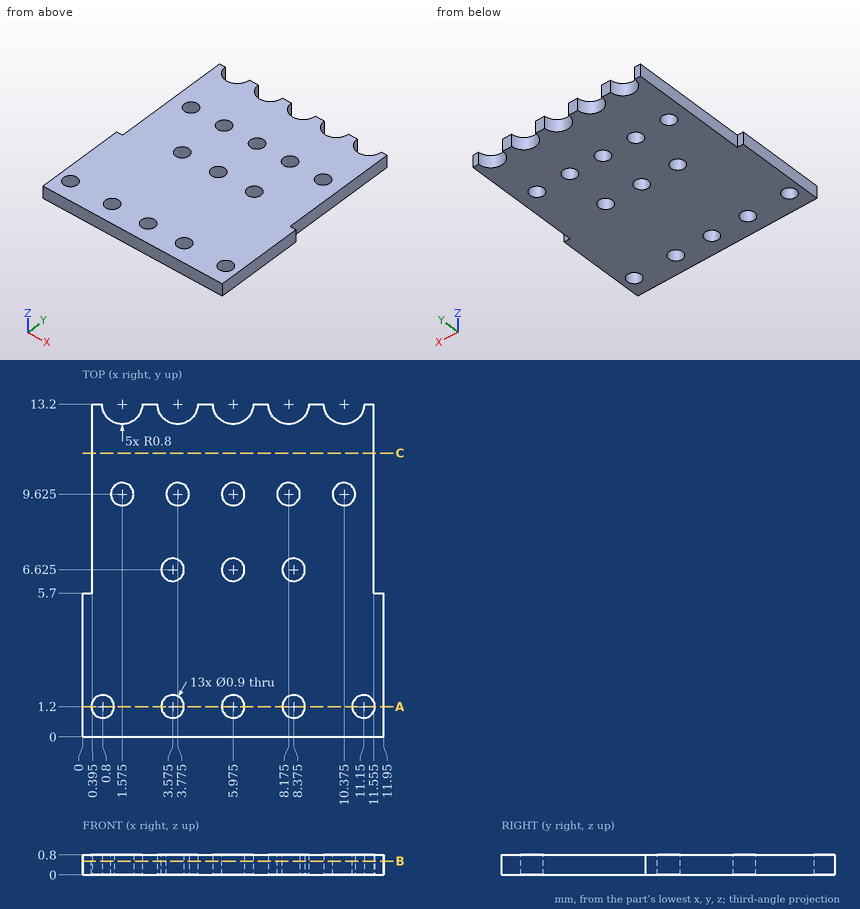
Could you check a few things on this drawing? It's one solid part, dimensions in mm from its lowest x, y, z. Round coordinates to 2 decimals unless told otherwise and drop trailing zeros. Order: outer loops, then holes, each group sorted by start corner. A loop starts at its lowest first (then second) coordinate and runs counter-clockwise, first axis right, second up. Notation, with made-up numbers: M -14,43.25 L -2,43.25 A19 ccw -2,51.25 Z; hole C 19.5,37 d11. An arc over 180 degrees is marked long. Return JSON: item names as keys, results as strings. Group by question number.
1. Please list where these lines run through material, in increasing order: probe 1 along Y at (x, z) = (6, 0.3); probe 2 along Y at (x, z) = (3.25, 0.35); probe 3 along X at (y, z) = (6.25, 0.2) (3 decimals).
2. If we section it at A-A on y = 1.2: List the corners of the cut face in (x, z) for me (3 decimals), then the cut area to 3 significant figures.
3. If we section it at B-B on z = 0.55: State how many separate pieces and enclosed holes the cut face has, then the cut area to 3 significant figures.
4. If we section it at C-C on y = 11.25: List the corners of the cut face in (x, z) for me (3 decimals).
Reply:
{
 "1": {"probe 1": "0 to 0.75, 1.65 to 6.18, 7.07 to 9.18, 10.07 to 12.4", "probe 2": "0 to 0.89, 1.51 to 6.31, 6.94 to 12.6", "probe 3": "0.395 to 3.326, 3.824 to 5.726, 6.224 to 8.126, 8.624 to 11.555"},
 "2": {"outline": "M 0,0 L 0.35,0 L 0.35,0.8 L 0,0.8 Z; M 1.25,0 L 3.125,0 L 3.125,0.8 L 1.25,0.8 Z; M 4.025,0 L 5.525,0 L 5.525,0.8 L 4.025,0.8 Z; M 6.425,0 L 7.925,0 L 7.925,0.8 L 6.425,0.8 Z; M 8.825,0 L 10.7,0 L 10.7,0.8 L 8.825,0.8 Z; M 11.6,0 L 11.95,0 L 11.95,0.8 L 11.6,0.8 Z", "area": "5.96 mm^2"},
 "3": {"separate pieces": "1", "enclosed holes": "13", "area": "139 mm^2"},
 "4": {"outline": "M 0.395,0 L 11.555,0 L 11.555,0.8 L 0.395,0.8 Z"}
}
